For this review, take the finished solid that the model builds, in its own axes (mm). Face numbers are marked on the shaded views. A direction names the side the tool comes from. Coordinates: 2 decimals unless noted, no trailing zeros. Write each loop counter-clockwise with the first axis right and the second up, starting at its lowest first coordinate (ties: lowest second). Pieces come first, ordered by that corner, then holes. Notation, with made-up numbers: (61, 79.25) -> (100, 79.25) arc R9 ccw to (100, 90.25) -> close; hole circle Ø11 at (30, 5). An arc over 180 degrees is marked (long way). One line per item, written item: value. Start each with the question number.
1) Add section B-B (x = 16.5). State the section outline as (y, z) points.
2) Add section A-A (y = 23). State the section outline as (x, z) points.
3) Add section D-D (z = -8). State how many separate pieces and enclosed holes the cut face has, and give its area (3 significant figures).
4) For pin 1 Ø1.5 at (x, z) = (16, -7) entering from -Y; pin 2 Ø2.5 at (x, z) = (16, -9.5) entering from +Y; pin 3 Ø4.5 at (x, y) = (36, 36.5) entering from -Z, all flat-tipped, find the tip position at first contact; note any pin that passes through.
5) Mouldability with a two-part tool opening along Z and no side actions: class the marked faces 1, 2 and 3 as released by +Z, released by -Z, zero draft, split by the parting line, or undercut.
6) Machinability: for the marked faces 4, 5 and 6, which of the approach directions +Z, -Z, +X, -X, +Y, -Y give a long, thin tool a straight path to every point of the face, cutting with its end or side? Answer none if there is none.
7) For probe 1 along X at (y, z) = (18.5, -6.5); probe 2 along Y at (x, z) = (34.55, -8); probe 3 along Y at (x, z) = (34.1, -8), list the stretches that pass through material, from the lowest coordinate up. Write a range as from..to.
8) Add section C-C (y = 16.5). State the section outline as (x, z) points, and give its area (3 significant figures).
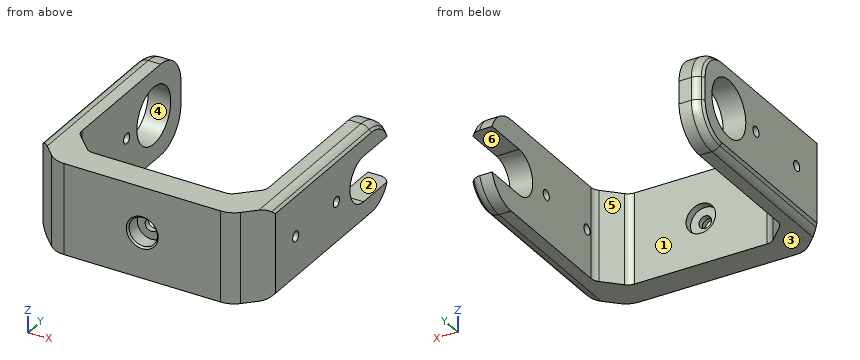
from build123d import *

# Parameters (mm, degrees)
SKETCH1_W           = 33
SKETCH1_H           = 16
SKETCH1_R           = 2.5
BOSS_EXTRUDE1_DEPTH = 2.7
SKETCH2_W           = 33
SKETCH2_H           = 16
SKETCH2_R           = 1.1
BOSS_EXTRUDE2_DEPTH = 2.3
SKETCH4_W           = 16
SKETCH4_H           = 39
SKETCH4_R           = 5
BOSS_EXTRUDE3_DEPTH = 4
BOSS_EXTRUDE4_DEPTH = 4
FILLET1_R           = 6
CHAMFER1_SIZE       = 4
SKETCH6_R           = 0.9
CUT_EXTRUDE1_DEPTH  = 59.804761712
CHAMFER2_SIZE       = 1
FILLET3_R           = 2
SKETCH7_R           = 2.6
CUT_EXTRUDE2_DEPTH  = 1.3
FILLET4_R           = 2
CHAMFER3_SIZE       = 5
FILLET7_R           = 4
CHAMFER4_SIZE       = 0.3


with BuildPart() as part:
    # Sketch1 → Boss-Extrude1 (new body)
    with BuildSketch(Plane(origin=(0, 0, 0), x_dir=(1, 0, 0), z_dir=(0, 1, 0))):
        with Locations((16.5, 8)):
            Rectangle(SKETCH1_W, SKETCH1_H)
        with Locations(Location((16.5, 8, 0), (0, 0, 90))):
            Circle(SKETCH1_R, mode=Mode.SUBTRACT)
    extrude(amount=BOSS_EXTRUDE1_DEPTH)

    # Sketch2 → Boss-Extrude2 (add)
    with BuildSketch(Plane(origin=(0, 2.7, 0), x_dir=(1, 0, 0), z_dir=(0, 1, 0))):
        with Locations((16.5, 8)):
            Rectangle(SKETCH2_W, SKETCH2_H)
        with Locations(Location((16.5, 8, 0), (0, 0, 270))):
            Circle(SKETCH2_R, mode=Mode.SUBTRACT)
    extrude(amount=BOSS_EXTRUDE2_DEPTH)

    # Sketch4 → Boss-Extrude3 (add)
    with BuildSketch(Plane.ZY):
        with Locations((-8, 19.5)):
            Rectangle(SKETCH4_W, SKETCH4_H)
        with Locations((-8, 31)):
            Circle(SKETCH4_R, mode=Mode.SUBTRACT)
    extrude(amount=BOSS_EXTRUDE3_DEPTH)

    # Sketch5 → Boss-Extrude4 (add)
    with BuildSketch(Plane(origin=(33, 0, 0), x_dir=(0, 0, -1), z_dir=(1, 0, 0))):
        with BuildLine():
            Line((0, 39), (4, 39))
            Line((4, 39), (4, 31))
            ThreePointArc((4, 31), (8, 27), (12, 31))
            Line((12, 31), (12, 39))
            Line((12, 39), (16, 39))
            Line((16, 39), (16, 0))
            Line((16, 0), (0, 0))
            Line((0, 0), (0, 39))
        make_face()
    extrude(amount=BOSS_EXTRUDE4_DEPTH)

    # Fillet1
    # the kernel refuses this fillet: 6 mm, written as the material it takes off along each edge
    with BuildSketch(Plane(origin=(18.857864376, 39, -16), x_dir=(0, -1, 0), z_dir=(1, 0, 0))) as fillet1_piece_1:
        with BuildLine():
            CenterArc((5.656854249, -6), FILLET1_R, 90, 70.528779366)
            Line((0, -4), (-0.113137085, -3.96))
            ThreePointArc((-0.113137085, -3.96), (-0.12, -2), (-0.12, 0))
            Line((-0.12, 0), (0, 0.12))
            Line((0, 0.12), (5.656854249, 0.12))
            Line((5.656854249, 0.12), (5.656854249, 0))
        make_face()
    extrude(amount=32.284271247, mode=Mode.SUBTRACT)
    with BuildSketch(Plane(origin=(15, 39, -16), x_dir=(0, -1, 0), z_dir=(-1, 0, 0))) as fillet1_piece_2:
        with BuildLine():
            CenterArc((FILLET1_R, FILLET1_R), FILLET1_R, 180, 90)
            Line((0, FILLET1_R), (-FILLET1_R * 0.02, FILLET1_R))
            Line((-FILLET1_R * 0.02, FILLET1_R), (-FILLET1_R * 0.02, -FILLET1_R * 0.02))
            Line((-FILLET1_R * 0.02, -FILLET1_R * 0.02), (FILLET1_R, -FILLET1_R * 0.02))
            Line((FILLET1_R, -FILLET1_R * 0.02), (FILLET1_R, 0))
        make_face()
    extrude(amount=34, mode=Mode.SUBTRACT)
    with BuildSketch(Plane(origin=(18.857864376, 39, 0), x_dir=(0, -1, 0), z_dir=(1, 0, 0))) as fillet1_piece_3:
        with BuildLine():
            CenterArc((5.656854249, 6), FILLET1_R, 199.471220634, 70.528779366)
            Line((0, 4), (-0.113137085, 3.96))
            ThreePointArc((-0.113137085, 3.96), (-0.12, 2), (-0.12, 0))
            Line((-0.12, 0), (0, -0.12))
            Line((0, -0.12), (5.656854249, -0.12))
            Line((5.656854249, -0.12), (5.656854249, 0))
        make_face()
    extrude(amount=32.284271247, mode=Mode.SUBTRACT)
    with BuildSketch(Plane(origin=(15, 39, 0), x_dir=(0, -1, 0), z_dir=(-1, 0, 0))) as fillet1_piece_4:
        with BuildLine():
            CenterArc((FILLET1_R, -FILLET1_R), FILLET1_R, 90, 90)
            Line((0, -FILLET1_R), (-FILLET1_R * 0.02, -FILLET1_R))
            Line((-FILLET1_R * 0.02, -FILLET1_R), (-FILLET1_R * 0.02, FILLET1_R * 0.02))
            Line((-FILLET1_R * 0.02, FILLET1_R * 0.02), (FILLET1_R, FILLET1_R * 0.02))
            Line((FILLET1_R, FILLET1_R * 0.02), (FILLET1_R, 0))
        make_face()
    extrude(amount=34, mode=Mode.SUBTRACT)

    # Chamfer1
    chamfer1_edges = [part.edges().sort_by_distance(p)[0] for p in [
        (0, 5, -8),
        (33, 5, -8),
    ]]
    chamfer(chamfer1_edges, length=CHAMFER1_SIZE)

    # Sketch6 → Cut-Extrude1 (cut, through all)
    with BuildSketch(Plane.ZY.offset(4)):
        with Locations((-8, 23)):
            Circle(SKETCH6_R)
        with Locations((-8, 11)):
            Circle(SKETCH6_R)
    extrude(amount=-CUT_EXTRUDE1_DEPTH, mode=Mode.SUBTRACT)

    # Chamfer2
    chamfer2_edges = [part.edges().sort_by_distance(p)[0] for p in [
        (-4, 16.5, 0),
        (37, 16.671572875, -16),
        (-4, 16.5, -16),
        (37, 16.671572875, 0),
        (37, 36.807247366, -1.101020514),
        (37, 36.807247366, -14.898979486),
        (-4, 39, -8),
        (-4, 37.242640687, -1.757359313),
        (-4, 37.242640687, -14.242640687),
    ]]
    chamfer(chamfer2_edges, length=CHAMFER2_SIZE)

    # Fillet3
    fillet3_edges = [part.edges().sort_by_distance(p)[0] for p in [
        (36, 16.671572875, -16),
        (36, 16.671572875, 0),
        (-3, 16.5, -16),
        (-3, 37.242640687, -14.242640687),
        (-3, 16.5, 0),
        (-3, 37.242640687, -1.757359313),
        (36, 36.807247366, -14.898979486),
        (36, 36.807247366, -1.101020514),
        (-3, 39, -8),
    ]]
    fillet(fillet3_edges, radius=FILLET3_R)

    # Sketch7 → Cut-Extrude2 (cut)
    with BuildSketch(Plane(origin=(0, 5, 0), x_dir=(1, 0, 0), z_dir=(0, 1, 0))):
        with Locations(Location((16.5, 8, 0), (0, 0, 270))):
            Circle(SKETCH7_R)
    extrude(amount=-CUT_EXTRUDE2_DEPTH, mode=Mode.SUBTRACT)

    # Fillet4
    fillet4_edges = [part.edges().sort_by_distance(p)[0] for p in [
        (29, 5, -8),
        (33, 9, -8),
        (0, 9, -8),
        (4, 5, -8),
    ]]
    fillet(fillet4_edges, radius=FILLET4_R)

    # Chamfer3
    chamfer3_edges = [part.edges().sort_by_distance(p)[0] for p in [
        (37, 0, -8),
        (-4, 0, -8),
    ]]
    chamfer(chamfer3_edges, length=CHAMFER3_SIZE)

    # Fillet7
    fillet7_edges = [part.edges().sort_by_distance(p)[0] for p in [
        (1, 0, -8),
        (32, 0, -8),
    ]]
    fillet(fillet7_edges, radius=FILLET7_R)

    # Chamfer4
    chamfer4_edges = [part.edges().sort_by_distance(p)[0] for p in [
        (16.5, 0, -5.5),
    ]]
    chamfer(chamfer4_edges, length=CHAMFER4_SIZE)


solid = part.part
Numbers:
1. outline: (0, -16) -> (5, -16) -> (5, -10.6) -> (3.7, -10.6) -> (3.7, -9.1) -> (2.7, -9.1) -> (2.7, -10.5) -> (0.3, -10.5) -> (0, -10.8) -> close; (0, -5.2) -> (0.3, -5.5) -> (2.7, -5.5) -> (2.7, -6.9) -> (3.7, -6.9) -> (3.7, -5.4) -> (5, -5.4) -> (5, 0) -> (0, 0) -> close
2. outline: (-4, -15) -> (-3.59, -15.41) arc R2 ccw to (-2.17, -16) -> (0, -16) -> (0, -8.9) -> (-4, -8.9) -> close; (-4, -7.1) -> (0, -7.1) -> (0, 0) -> (-2.17, 0) arc R2 ccw to (-3.59, -0.59) -> (-4, -1) -> close; (33, -16) -> (35.17, -16) arc R2 ccw to (36.59, -15.41) -> (37, -15) -> (37, -8.9) -> (33, -8.9) -> close; (33, -7.1) -> (37, -7.1) -> (37, -1) -> (36.59, -0.59) arc R2 ccw to (35.17, 0) -> (33, 0) -> close
3. separate pieces: 7
3. enclosed holes: 0
3. area: 328 mm²
4. pin 1: y = 2.7
4. pin 2: y = 5
4. pin 3: z = -15.91
5. face 1: zero draft
5. face 2: undercut
5. face 3: released by -Z
6. face 4: -X
6. face 5: +Z, -Z, +Y
6. face 6: +X, +Y
7. probe 1: -4..0, 33..37
7. probe 2: 2.55..10.1, 11.9..22.1, 23.9..27
7. probe 3: 2.1..10.1, 11.9..22.1, 23.9..27
8. outline: (-4, -15) -> (-3.59, -15.41) arc R2 ccw to (-2.17, -16) -> (0, -16) -> (0, 0) -> (-2.17, 0) arc R2 ccw to (-3.59, -0.59) -> (-4, -1) -> close; (33, -16) -> (35.17, -16) arc R2 ccw to (36.59, -15.41) -> (37, -15) -> (37, -1) -> (36.59, -0.59) arc R2 ccw to (35.17, 0) -> (33, 0) -> close
8. area: 126 mm²
